from build123d import *

# Parameters (mm, degrees)
BOX046_W                     = 6
BOX046_H                     = 7
BOX046_DEPTH                 = 7.4
BOX045_W                     = 7
BOX045_H                     = 12
BOX045_DEPTH                 = 4
CHAMFER_SIZE                 = 1
CHAMFER_PLACEMENT_ANGLE      = 90
FUSION002026_PLACEMENT_ANGLE = 90


with BuildPart() as cubo046:
    # Box046 → Box046 (new body)
    with BuildSketch(Plane(origin=(-13, -15, 2.5), x_dir=(1, 0, 0), z_dir=(0, 0, 1))):
        with Locations((3, 3.5)):
            Rectangle(BOX046_W, BOX046_H)
    extrude(amount=BOX046_DEPTH)


with BuildPart() as fusion002026:
    # Box045 → Box045 (new body)
    with BuildSketch(Plane(origin=(-13, -7, 2), x_dir=(1, 0, 0), z_dir=(0, 0, -1))):
        with Locations((3.5, 6)):
            Rectangle(BOX045_W, BOX045_H)
    extrude(amount=BOX045_DEPTH)

    # Chamfer
    chamfer_edges = [fusion002026.edges().sort_by_distance(p)[0] for p in [
        (-13, -13, -2),
    ]]
    chamfer(chamfer_edges, length=CHAMFER_SIZE)


with BuildPart() as fusion002026_1:
    # Chamfer placement: moved
    add(fusion002026.part.moved(Location((-23.5, -2, 0.5))).rotate(Axis((-23.5, -2, 0.5), (0, 0, 1)), CHAMFER_PLACEMENT_ANGLE))

    # Fusion002026: union Cubo046
    add(cubo046.part)


with BuildPart() as fusion002026_2:
    # Fusion002026 placement: moved
    add(fusion002026_1.part.moved(Location((-44, 70, 34.3))).rotate(Axis((-44, 70, 34.3), (0, 0, 1)), FUSION002026_PLACEMENT_ANGLE))


solid = fusion002026_2.part
Read the model definition and answer for the solid it produces. Units are mm, in the model's axes. A direction names the side the tool comes from. Give positions to 0.01 mm unless a question says otherwise; leave off trailing zeros. Write each loop counter-clockwise with the first axis right and the second up, starting at its lowest first coordinate (ties: lowest second). Pieces come first, ordered by that corner, then holes. Notation, with made-up numbers: M 61.25,4 L 102.25,4 A12 cw 102.25,9 Z; hole C 54,45 d1. An arc over 180 degrees is marked long. One line per item, written item: value. Start each with the question number.
(1) Find section C-C (z = 39.5). Determine the outline of the cut face in (x, y).
(2) Flat-ended cylindrical pins translate along their axes: pin 1 Ø3 at (x, z) = (-33.5, 43) entering from +Y; pin 2 Ø1 at (x, y) = (-31, 54.5) entering from +Z. Find the tip coordinate at first contact, or state that the pin passes through.
(3) Find section B-B (y = 56.75). Determine the outline of the cut face in (x, z), plus the area to 3 significant figures.
(4) Find the intervals of material crossed by line 1 (Y direction, x = -34.5, z = 39); line 2 (Z direction, x = -35.5, y = 56); line 3 (X direction, y = 64.5, z = 33.5), in increasing order.
(5) A tool of negligible diameter and unlimited length cuts with its end or side. For faces 1 (the flat face through (-32, 57, 40)), 2 (the flat face through (-33, 60, 44.2)), 3 (the flat face through (-32, 63, 40)), from which of +Z, -Z, +X, -X, +Y, -Y can it reach the whole face along a straight path? Write none if from no direction.
(6) Find section A-A (x = -32.5). Determine the outline of the cut face in (y, z).
Results below:
1. outline: M -36,57 L -29,57 L -29,63 L -36,63 Z
2. pin 1: stops at y = 63
2. pin 2: stops at z = 36.8
3. outline: M -36,32.8 L -30,32.8 L -29,33.8 L -29,36.8 L -36,36.8 Z
3. area: 27.5 mm^2
4. line 1: y = 57 to 63
4. line 2: z = 32.8 to 36.8
4. line 3: x = -36 to -29.3
5. face 1: +Z, +X, -X, -Y
5. face 2: +Z, +X, -X, +Y, -Y
5. face 3: +Z, +X, -X, +Y
6. outline: M 53.5,32.8 L 65.5,32.8 L 65.5,36.8 L 63,36.8 L 63,44.2 L 57,44.2 L 57,36.8 L 53.5,36.8 Z
